CAD build for the part. Positions are in the model's coordinates, mm. Give positions to 0.01 mm unless a question says otherwise; leave off trailing zeros. Write each loop counter-clockwise with the first axis right and the second up, starting at its lowest first coordinate (ties: lowest second). Pieces come first, ordered by that corner, then holes. Notation, with made-up numbers: (54, 19) - (82, 19) arc R10 cw to (82, 37) - close; hole circle Ø6 at (11.25, 28.5). An arc over 180 degrees is marked (long way). Answer as a JSON object with one key per item and string values.
from build123d import *

# Parameters (mm, degrees)
SKETCH_1_R               = 25
EXTRUDE_1_DEPTH          = 100
FILLET_1_R               = 25
CUT_EXTRUDE_2_DEPTH      = 200
CUT_EXTRUDE_2_DEPTH_BACK = 200
SKETCH_2_OUTSIDE_W       = 76.494
SKETCH_2_OUTSIDE_H       = 126.494
SKETCH_2_OUTSIDE_W_2     = 35
SKETCH_2_OUTSIDE_H_2     = 100
SKETCH_3_R               = 7.5
CUT_EXTRUDE_3_DEPTH      = 109.857705285


with BuildPart() as part:
    # Sketch 1 → Extrude 1 (new body)
    with BuildSketch(Plane(origin=(0, 0, 0), x_dir=(1, 0, 0), z_dir=(0, 1, 0))):
        with Locations(Location((0, 0, 0), (0, 0, 270))):
            Circle(SKETCH_1_R)
    extrude(amount=EXTRUDE_1_DEPTH)

    # Fillet 1
    fillet_1_edges = [part.edges().sort_by_distance(p)[0] for p in [
        (0, 0, -25),
        (0, 100, -25),
    ]]
    fillet(fillet_1_edges, radius=FILLET_1_R)

    # Sketch 2 outside → Cut-Extrude 2 (cut, two sides: drawn at the far end of the back side and taken through both)
    with BuildSketch(Plane.XY.offset(-CUT_EXTRUDE_2_DEPTH_BACK)):
        with Locations((0, 50)):
            Rectangle(SKETCH_2_OUTSIDE_W, SKETCH_2_OUTSIDE_H)
        with Locations((0, 50)):
            Rectangle(SKETCH_2_OUTSIDE_W_2, SKETCH_2_OUTSIDE_H_2, mode=Mode.SUBTRACT)
    extrude(amount=CUT_EXTRUDE_2_DEPTH + CUT_EXTRUDE_2_DEPTH_BACK, mode=Mode.SUBTRACT)

    # Sketch 3 → Cut-Extrude 3 (cut, through all)
    with BuildSketch(Plane.ZY.offset(17.5)):
        with Locations(Location((0, 75, 0), (0, 0, 270))):
            Circle(SKETCH_3_R)
        with Locations(Location((0, 25, 0), (0, 0, 270))):
            Circle(SKETCH_3_R)
    extrude(amount=-CUT_EXTRUDE_3_DEPTH, mode=Mode.SUBTRACT)


solid = part.part
(1) Flat gauge pins, fed straight in: P1, Ø1.5, axis at x = 8.5, z = 14.5, coming from the -Y side; P2, Ø10, axis at x = -6.5, z = -18, coming from the -Y side; P3, Ø3, axis at x = 4, y = 31.5, coming from the +Z side; P4, Ø12, axis at y = 25, z = 0, coming from the +X side. Where does each tip first touch, or does it go through?
Answer key:
{"P1": "stops at y = 5.84", "P2": "stops at y = 4.38", "P3": "stops at z = 24.87", "P4": "passes through"}
(2) Saw through at B-B, the plane x = 15. Give the cut face in (y, z).
Answer key:
{"outline": "(25, -20) - (75, -20) arc R20 ccw to (75, 20) - (25, 20) arc R20 ccw to start; hole circle Ø15 at (25, 0); hole circle Ø15 at (75, 0)"}
(3) Pull direction Z, two halves, no side cores. Call faces 1 (the face through (0, 50, -25)), 2 (the face through (0, 50, 25)), 3 (the face through (-0.2, 80.5, 5.1)), 4 (the face through (-0.245, 32.493, 0.33)): pulls with the +Z half, pulls with the -Z half, needs draft (parallel to the pull), parting line crosses it, or undercut.
Answer key:
{"face 1": "pulls with the -Z half", "face 2": "pulls with the +Z half", "face 3": "undercut", "face 4": "undercut"}
(4) Saw through at D-D, the plane z = 20. Give the cut face in (x, y), and give its area (3 significant figures).
Answer key:
{"outline": "(-15, 25) arc R15 ccw to (15, 25) - (15, 75) arc R15 ccw to (-15, 75) - close", "area": "2,210 mm²"}
(5) Saw through at C-C, the plane y = 71. Give the cut face in (x, z).
Answer key:
{"outline": "(-17.5, -17.85) arc R25 ccw to (17.5, -17.85) - (17.5, -6.34) - (-17.5, -6.34) - close; (-17.5, 6.34) - (17.5, 6.34) - (17.5, 17.85) arc R25 ccw to (-17.5, 17.85) - close"}
(6) Saw through at A-A, the plane z = 0. Give the cut face in (x, y).
Answer key:
{"outline": "(-17.5, 7.15) arc R25 ccw to (17.5, 7.15) - (17.5, 17.5) - (-17.5, 17.5) - close; (-17.5, 32.5) - (17.5, 32.5) - (17.5, 67.5) - (-17.5, 67.5) - close; (-17.5, 82.5) - (17.5, 82.5) - (17.5, 92.85) arc R25 ccw to (-17.5, 92.85) - close"}
(7) Probe L1, parallel to Y at x = 10.5, z = -4; L2, parallel to Z at x = 4.5, y = 31; L3, parallel to Y at x = 12.5, z = -4. List the from-to ranges inside material, lowest first. Write a range as [from, to].
Answer key:
{"L1": "y = [2.67, 18.66], [31.34, 68.66], [81.34, 97.33]", "L2": "z = [-24.59, -4.5], [4.5, 24.59]", "L3": "y = [3.72, 18.66], [31.34, 68.66], [81.34, 96.28]"}
